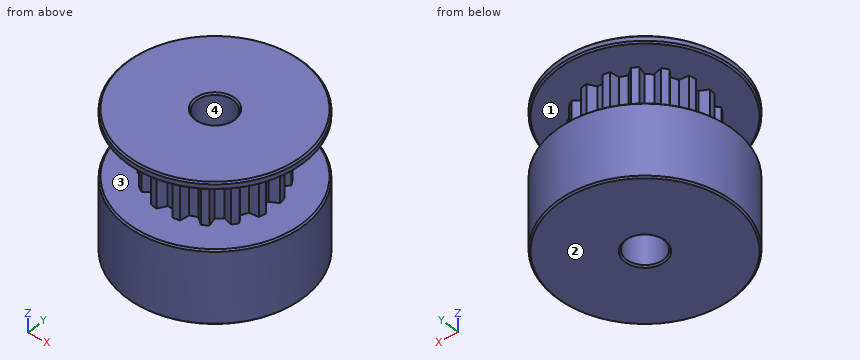
from build123d import *

# Parameters (mm, degrees)
ESQUISSE1_R                  = 8
BOSS_EXTRU_1_DEPTH           = 8
ENL_V_MAT_EXTRU_1_DEPTH      = 9
R_P_TITION_CIRCULAIRE1_COUNT = 16
ESQUISSE3_R                  = 12
BOSS_EXTRU_2_DEPTH           = 10
ESQUISSE4_R                  = 12
BOSS_EXTRU_3_DEPTH           = 1
CHANFREIN1_SIZE              = 0.2
ESQUISSE5_R                  = 2.5
ENL_V_MAT_EXTRU_2_DEPTH      = 20
CHANFREIN2_SIZE              = 0.2


with BuildPart() as part:
    # Esquisse1 → Boss.-Extru.1 (new body)
    with BuildSketch(Plane.XY):
        Circle(ESQUISSE1_R)
    extrude(amount=BOSS_EXTRU_1_DEPTH)

    # Esquisse2 → Enlèv. mat.-Extru.1 (cut, through all)
    with BuildSketch(Plane.XY.offset(8)):
        with BuildLine():
            Line((-1.120772376, 7.921102782), (-0.5, 6.845893487))
            Line((-0.5, 6.845893487), (0.5, 6.845893487))
            Line((0.5, 6.845893487), (1.120772376, 7.921102782))
            ThreePointArc((1.120772376, 7.921102782), (0, 8), (-1.120772376, 7.921102782))
        make_face()
    enl_v_mat_extru_1 = extrude(amount=-ENL_V_MAT_EXTRU_1_DEPTH, mode=Mode.SUBTRACT)

    # Répétition circulaire1: Enlèv. mat.-Extru.1 ×16 about axis
    r_p_tition_circulaire1_axis = Axis((0, 0, 0), (0, 0, 1))
    for i in range(1, R_P_TITION_CIRCULAIRE1_COUNT):
        add(enl_v_mat_extru_1.rotate(r_p_tition_circulaire1_axis, i * 360 / R_P_TITION_CIRCULAIRE1_COUNT), mode=Mode.SUBTRACT)

    # Esquisse3 → Boss.-Extru.2 (add)
    with BuildSketch(Plane(origin=(0, 0, 0), x_dir=(-1, 0, 0), z_dir=(0, 0, -1))):
        Circle(ESQUISSE3_R)
    extrude(amount=BOSS_EXTRU_2_DEPTH)

    # Esquisse4 → Boss.-Extru.3 (add)
    with BuildSketch(Plane.XY.offset(8)):
        Circle(ESQUISSE4_R)
    extrude(amount=BOSS_EXTRU_3_DEPTH)

    # Chanfrein1
    chanfrein1_edges = [part.edges().sort_by_distance(p)[0] for p in [
        (12, 0, 0),
        (12, 0, -10),
        (-12, 0, 8),
        (-12, 0, 9),
    ]]
    chamfer(chanfrein1_edges, length=CHANFREIN1_SIZE)

    # Esquisse5 → Enlèv. mat.-Extru.2 (cut, through all)
    with BuildSketch(Plane(origin=(0, 0, -10), x_dir=(-1, 0, 0), z_dir=(0, 0, -1))):
        Circle(ESQUISSE5_R)
    extrude(amount=-ENL_V_MAT_EXTRU_2_DEPTH, mode=Mode.SUBTRACT)

    # Chanfrein2
    chanfrein2_edges = [part.edges().sort_by_distance(p)[0] for p in [
        (2.5, 0, 9),
        (2.5, 0, -10),
    ]]
    chamfer(chanfrein2_edges, length=CHANFREIN2_SIZE)


solid = part.part
CAD build for the part. Positions are in the model's coordinates, mm. Face numbers are marked on the shaded views. Round coordinates to 2 decimals unless told otherwise and drop trailing zeros. Write each loop counter-clockwise with the first axis right and the second up, starting at its lowest first coordinate (ties: lowest second). Pieces come first, ordered by that corner, then holes.
(1) Probe line 1 along Z through (x, y) = (-8.5, -2); line 2 along Y through (x, z) = (0, 1); line 3 along Y through (x, z) = (-1, 7.75). List the from-to ranges inside material, lowest first.
(2) Drop flat-ended pins along their axis: P1, Ø8, axis at x = 0, y = 0, coming from the -Z side; P2, Ø3, axis at x = 3.5, z = -1.5, coming from the +Y side; P3, Ø1.5, axis at x = 6, z = -2.5, coming from the -Y side; P4, Ø1.1, axis at y = 0, z = 5.5, coming from the +X side. Give the stop position or say it passes through.
(3) Slice it at A-A, the plane x = 0. Write the cut outline in (y, z), and give its area (3 significant figures).
(4) Mould opens along Z. For the marked faces 1, 2, 3 and 4 say: pulls with the +Z half, pulls with the -Z half, needs draft (parallel to the pull), parting line crosses it, or undercut.
From the geometry:
1. line 1: z = -10 to 0, 8 to 9
1. line 2: y = -6.85 to -2.5, 2.5 to 6.85
1. line 3: y = -7.71 to -2.29, 2.29 to 7.71
2. P1: stops at z = -10
2. P2: stops at y = 11.83
2. P3: stops at y = -10.79
2. P4: stops at x = 6.93
3. outline: (-12, -9.8) - (-11.8, -10) - (-2.7, -10) - (-2.5, -9.8) - (-2.5, 8.8) - (-2.7, 9) - (-11.8, 9) - (-12, 8.8) - (-12, 8.2) - (-11.8, 8) - (-6.85, 8) - (-6.85, 0) - (-11.8, 0) - (-12, -0.2) - close; (2.5, -9.8) - (2.7, -10) - (11.8, -10) - (12, -9.8) - (12, -0.2) - (11.8, 0) - (6.85, 0) - (6.85, 8) - (11.8, 8) - (12, 8.2) - (12, 8.8) - (11.8, 9) - (2.7, 9) - (2.5, 8.8) - close
3. area: 278 mm2
4. face 1: undercut
4. face 2: pulls with the -Z half
4. face 3: undercut
4. face 4: needs draft
